Can you work these out from the model? Positions are in its coordinate system, mm. A direction names the side the tool comes from. Round coordinates to 2 decimals unless told otherwise and drop trailing zeros. Order: outer loops, then holes, each group sorted by start corner. A loop starts at its lowest first (then second) coordinate and runs counter-clockwise, first axis right, second up. Notation, with made-up numbers: M 88,40.25 L 99,40.25 A27 ccw 99,68.25 Z; hole C 28.25,41.5 d3. An arc over 180 degrees is marked long. One line per question, with ' | ' between items.
```python
from build123d import *

# Parameters (mm, degrees)
F0_R     = 22
F0_R_2   = 16
F1_DEPTH = 1.5
F2_R     = 19.9
F2_R_2   = 18
F3_DEPTH = 3


# Not quite as in the source:
# - a feature names something its author has since deleted; it is built from what else it names


with BuildPart() as f1:
    # F0 (on Front) → F1 (new body)
    with BuildSketch(Plane.XZ):
        Circle(F0_R)
        Circle(F0_R_2, mode=Mode.SUBTRACT)
    extrude(amount=F1_DEPTH)

    # F2 (on face) → F3 (join)
    with BuildSketch(Plane.XZ.offset(1.5)):
        Circle(F2_R)
        Circle(F2_R_2, mode=Mode.SUBTRACT)
    extrude(amount=F3_DEPTH)


solid = f1.part
```
(1) If we section it at A-A on x = 0: Please give me the cut outline in (y, z), plus the area to 3 significant figures.
Final values:
outline: M -4.5,-19.9 L -1.5,-19.9 L -1.5,-22 L 0,-22 L 0,-16 L -1.5,-16 L -1.5,-18 L -4.5,-18 Z; M -4.5,18 L -1.5,18 L -1.5,16 L 0,16 L 0,22 L -1.5,22 L -1.5,19.9 L -4.5,19.9 Z | area: 29.4 mm^2
(2) If we section it at C-C on y = -0.8: Please give me the cut outline in (x, z).
Final values:
outline: C 0,0 d44; hole C 0,0 d32
(3) Thinking about a two-plate mould opening in X: for faces 1 (the cylindrical face through (-2.343, -2.979, 17.847)), 2 (the flat face through (-5, -1.5, -19.5)), 3 (the cylindrical face through (-15.8, -3, -12.1)), which applies, released by +X, released by -X, zero draft, split by the parting line, or undercut?
Final values:
face 1: undercut | face 2: zero draft | face 3: split by the parting line
(4) On a 3-axis mill with a long thin cutter (end or side, diameter ignored), from which of +Z, -Z, +X, -X, +Y, -Y can I reach the whole of each face in a straight line? I mean faces 4 (the cylindrical face through (-4.769, -0.74, -21.477)), 5 (the flat face through (-12, -1.5, -11)). Say none if no direction works.
Final values:
face 4: +Y, -Y | face 5: -Y
(5) Please list where these lines run through material, in increasing order: probe 1 along Z at (x, y) = (0, -2.9); probe 2 along Z at (x, y) = (0, -1.05); probe 3 along Y at (x, z) = (11, -18.5). Write a range as [from, to].
Final values:
probe 1: [-19.9, -18], [18, 19.9] | probe 2: [-22, -16], [16, 22] | probe 3: [-1.5, 0]
(6) If we section it at B-B on z = 15.5: Please give me the cut outline in (x, y).
Final values:
outline: M -15.61,-1.5 L -12.48,-1.5 L -12.48,-4.5 L -9.15,-4.5 L -9.15,-1.5 L -3.97,-1.5 L -3.97,0 L -15.61,0 Z; M 3.97,-1.5 L 9.15,-1.5 L 9.15,-4.5 L 12.48,-4.5 L 12.48,-1.5 L 15.61,-1.5 L 15.61,0 L 3.97,0 Z
